```python
from build123d import *

# Parameters (mm, degrees)
F1_W     = 20
F1_H     = 25
F2_DEPTH = 3
F3_R     = 1.5
F4_DEPTH = 12
F0_R     = 0.5


with BuildPart() as f2:
    # F1 (on Top) → F2 (new body)
    with BuildSketch(Plane.XY):
        Rectangle(F1_W, F1_H)
    extrude(amount=F2_DEPTH)

    # F3 (on face) → F4 (join)
    with BuildSketch(Plane(origin=(0, 0, 0), x_dir=(1, 0, 0), z_dir=(0, 0, -1))):
        Circle(F3_R)
    extrude(amount=F4_DEPTH)

    # F0
    f0_edges = [f2.edges().sort_by_distance(p)[0] for p in [
        (-1.5, 0, -12),
    ]]
    fillet(f0_edges, radius=F0_R)


solid = f2.part
```
For this review, take the finished solid that the model builds, in its own axes (mm). A direction names the side the tool comes from. Round coordinates to 2 decimals unless told otherwise and drop trailing zeros. Loops run counter-clockwise (first coordinate to the right, second up) from the corner with the lowest first, then second, coordinate; pieces in that order, holes last.
(1) We need section B-B (y = 0). Give the boundary of the cut face in (x, z).
Returned:
outline: (-10, 0) - (-1.5, 0) - (-1.5, -11.5) arc R0.5 ccw to (-1, -12) - (1, -12) arc R0.5 ccw to (1.5, -11.5) - (1.5, 0) - (10, 0) - (10, 3) - (-10, 3) - close
(2) Tool access review of faces 1 (the flat face through (0, -12.5, 1)), 2 (the cylindrical face through (-1.5, -0.07, -5.67)): name each direction out of +Z, -Z, +X, -X, +Y, -Y from which nothing blocks a thin tool from reaching the whole face with its end or side.
Returned:
face 1: +Z, -Z, +X, -X, -Y
face 2: -Z
(3) Clearance check with flat-ended pins moving along their axes: P1, Ø10, axis at x = 6.5, y = 7, coming from the -Z side; P2, Ø8, axis at y = 3, z = -7.5, coming from the +X side; P3, Ø4, axis at x = 1.5, z = -1, coming from the +Y side. State where each tip first meets the part, or that it passes through.
Returned:
P1: stops at z = 0
P2: stops at x = 1.5
P3: stops at y = 12.5
(4) We need section D-D (y = -2.75). Give the boundary of the cut face in (x, z), plus the area to 3 significant figures.
Returned:
outline: (-10, 0) - (10, 0) - (10, 3) - (-10, 3) - close
area: 60.0 mm2
(5) We need section A-A (x = 0). Give the boundary of the cut face in (y, z).
Returned:
outline: (-12.5, 0) - (-1.5, 0) - (-1.5, -11.5) arc R0.5 ccw to (-1, -12) - (1, -12) arc R0.5 ccw to (1.5, -11.5) - (1.5, 0) - (12.5, 0) - (12.5, 3) - (-12.5, 3) - close
(6) We need section C-C (z = -2.75). Give the boundary of the cut face in (x, y), plus the area to 3 significant figures.
Returned:
outline: circle Ø3 at (0, 0)
area: 7.07 mm2
(7) Wall thickness on line 1 along Z through (x, y) = (-7, -0.25); line 2 along Z through (x, y) = (1, -0.5); line 3 along Y through (x, z) = (1, -7.75): over which ranges is each line inside the solid? List them lowest first.
Returned:
line 1: z = 0 to 3
line 2: z = -11.99 to 3
line 3: y = -1.12 to 1.12
